For this review, take the finished solid that the model builds, in its own axes (mm). A direction names the side the tool comes from. Round coordinates to 2 decimals unless told otherwise and drop trailing zeros. Order: outer loops, then holes, each group sorted by start corner. A loop starts at its lowest first (then second) coordinate and runs counter-clockwise, first axis right, second up. Notation, with made-up numbers: (84.25, -17) -> (113.25, -17) arc R14 ccw to (113.25, -8) -> close; hole circle Ø7 at (76, -11). An arc over 180 degrees is marked (long way). Answer in a Markdown table with one row per item.
```python
from build123d import *

# Parameters (mm, degrees)
BOSS_EXTRUDE1_DEPTH = 2
SKETCH2_W           = 3
SKETCH2_H           = 52
BOSS_EXTRUDE2_DEPTH = 50
SKETCH3_R           = 4
CUT_EXTRUDE1_DEPTH  = 90


with BuildPart() as part:
    # Sketch1 → Boss-Extrude1 (new body)
    with BuildSketch(Plane(origin=(0, 0, 0), x_dir=(1, 0, 0), z_dir=(0, 1, 0))):
        with BuildLine():
            Line((-32.5, 28), (-27.204017471, 28))
            ThreePointArc((-27.204017471, 28), (-25.789803909, 27.414213562), (-25.204017471, 26))
            Line((-25.204017471, 26), (-25.204017471, -26))
            ThreePointArc((-25.204017471, -26), (-25.789803909, -27.414213562), (-27.204017471, -28))
            Line((-27.204017471, -28), (-32.5, -28))
            ThreePointArc((-32.5, -28), (-33.914213562, -28.585786438), (-34.5, -30))
            Line((-34.5, -30), (-34.5, -48))
            Line((-34.5, -48), (34.5, -48))
            Line((34.5, -48), (34.5, -30))
            ThreePointArc((34.5, -30), (33.914213562, -28.585786438), (32.5, -28))
            Line((32.5, -28), (27.204017471, -28))
            ThreePointArc((27.204017471, -28), (25.789803909, -27.414213562), (25.204017471, -26))
            Line((25.204017471, -26), (25.204017471, 26))
            ThreePointArc((25.204017471, 26), (25.789803909, 27.414213562), (27.204017471, 28))
            Line((27.204017471, 28), (32.5, 28))
            ThreePointArc((32.5, 28), (33.914213562, 28.585786438), (34.5, 30))
            Line((34.5, 30), (34.5, 48))
            Line((34.5, 48), (-34.5, 48))
            Line((-34.5, 48), (-34.5, 30))
            ThreePointArc((-34.5, 30), (-33.914213562, 28.585786438), (-32.5, 28))
        make_face()
        with BuildLine():
            Line((-26.353730012, 40.955917197), (-26.353730012, 38.634748977))
            ThreePointArc((-26.353730012, 38.634748977), (-27.768725827, 37.219753162), (-29.183721642, 38.634748977))
            Line((-29.183721642, 38.634748977), (-29.183721642, 40.955917197))
            ThreePointArc((-29.183721642, 40.955917197), (-27.768725827, 42.370913012), (-26.353730012, 40.955917197))
        make_face(mode=Mode.SUBTRACT)
        with BuildLine():
            Line((26.353730012, 40.955917197), (26.353730012, 38.634748977))
            ThreePointArc((26.353730012, 38.634748977), (27.768725827, 37.219753162), (29.183721642, 38.634748977))
            Line((29.183721642, 38.634748977), (29.183721642, 40.955917197))
            ThreePointArc((29.183721642, 40.955917197), (27.768725827, 42.370913012), (26.353730012, 40.955917197))
        make_face(mode=Mode.SUBTRACT)
        with BuildLine():
            Line((-26.353730012, -40.955917197), (-26.353730012, -38.634748977))
            ThreePointArc((-26.353730012, -38.634748977), (-27.768725827, -37.219753162), (-29.183721642, -38.634748977))
            Line((-29.183721642, -38.634748977), (-29.183721642, -40.955917197))
            ThreePointArc((-29.183721642, -40.955917197), (-27.768725827, -42.370913012), (-26.353730012, -40.955917197))
        make_face(mode=Mode.SUBTRACT)
        with BuildLine():
            Line((26.353730012, -40.955917197), (26.353730012, -38.634748977))
            ThreePointArc((26.353730012, -38.634748977), (27.768725827, -37.219753162), (29.183721642, -38.634748977))
            Line((29.183721642, -38.634748977), (29.183721642, -40.955917197))
            ThreePointArc((29.183721642, -40.955917197), (27.768725827, -42.370913012), (26.353730012, -40.955917197))
        make_face(mode=Mode.SUBTRACT)
    extrude(amount=BOSS_EXTRUDE1_DEPTH)

    # Sketch2 → Boss-Extrude2 (add)
    with BuildSketch(Plane(origin=(0, 2, 0), x_dir=(1, 0, 0), z_dir=(0, 1, 0))):
        with Locations((-23.704017471, 0)):
            Rectangle(SKETCH2_W, SKETCH2_H)
        with Locations((23.704017471, 0)):
            Rectangle(SKETCH2_W, SKETCH2_H)
    extrude(amount=BOSS_EXTRUDE2_DEPTH)

    # Sketch3 → Cut-Extrude1 (cut)
    with BuildSketch(Plane.ZY.offset(25.204017471)):
        with BuildLine():
            Line((-26, 52), (-26, 32))
            ThreePointArc((-26, 32), (-20.142135624, 46.142135624), (-6, 52))
            Line((-6, 52), (-26, 52))
        make_face()
        with BuildLine():
            ThreePointArc((6, 52), (20.142135624, 46.142135624), (26, 32))
            Line((26, 32), (26, 52))
            Line((26, 52), (6, 52))
        make_face()
        with Locations((0, 40)):
            Circle(SKETCH3_R)
    extrude(amount=-CUT_EXTRUDE1_DEPTH, mode=Mode.SUBTRACT)


solid = part.part
```
Q1. Take a section at C-C, the plane y = 40. Write out the cut boundary in (x, z), then the cut area to 3 significant figures.
Answer key:
| item | result |
|---|---|
| outline | (-25.2, -24.33) -> (-22.2, -24.33) -> (-22.2, -4) -> (-25.2, -4) -> close; (-25.2, 4) -> (-22.2, 4) -> (-22.2, 24.33) -> (-25.2, 24.33) -> close; (22.2, -24.33) -> (25.2, -24.33) -> (25.2, -4) -> (22.2, -4) -> close; (22.2, 4) -> (25.2, 4) -> (25.2, 24.33) -> (22.2, 24.33) -> close |
| area | 244 mm^2 |
Q2. Take a section at A-A, the plane z = 0. Write out the cut boundary in (x, y), then the cut area to 3 significant figures.
Answer key:
| item | result |
|---|---|
| outline | (-25.2, 0) -> (25.2, 0) -> (25.2, 36) -> (22.2, 36) -> (22.2, 2) -> (-22.2, 2) -> (-22.2, 36) -> (-25.2, 36) -> close; (-25.2, 44) -> (-22.2, 44) -> (-22.2, 52) -> (-25.2, 52) -> close; (22.2, 44) -> (25.2, 44) -> (25.2, 52) -> (22.2, 52) -> close |
| area | 353 mm^2 |
Q3. Clearance check with flat-ended pins moving along their axes: pin 1 Ø0.9 at (x, y) = (24, 11.5) entering from -Z; pin 2 Ø0.9 at (x, y) = (-23, 23) entering from +Z; pin 3 Ø12 at (x, z) = (-12, -19) entering from +Y; pin 4 Ø2 at (x, z) = (-27, 3.5) entering from -Y. State where each tip first meets the part, or that it passes through.
Answer key:
| item | result |
|---|---|
| pin 1 | stops at z = -26 |
| pin 2 | stops at z = 26 |
| pin 3 | stops at y = 2 |
| pin 4 | passes through |
Q4. The part is to be moulded in two halves that separate along X. For faces 1 (the face through (-30, 1, -28)), 2 (the face through (-27.8, 0.99, 42.37)), 3 (the face through (25.805, 0.986, 27.43)), say which applies: +X half, -X half, draft (parallel to the pull), parting line (faces both ways), or undercut.
Answer key:
| item | result |
|---|---|
| face 1 | draft |
| face 2 | undercut |
| face 3 | +X half |
Q5. Tool access review of faces 4 (the face through (29.184, 1, 40)), 5 (the face through (30, 1, 28)), 6 (the face through (-23.725, 46.297, 19.986)), 7 (the face through (-33.93, 0.99, -28.6)), 8 (the face through (-23.725, 43.966, -0.521)): name each direction out of +Z, -Z, +X, -X, +Y, -Y from which nothing blocks a thin tool from reaching the whole face with its end or side.
Answer key:
| item | result |
|---|---|
| face 4 | +Y, -Y |
| face 5 | +X, +Y, -Y |
| face 6 | +Z, +X, -X, +Y |
| face 7 | -X, +Y, -Y |
| face 8 | +X, -X |
Q6. Take a section at D-D, the plane z = 15. Write out the cut boundary in (x, y).
Answer key:
| item | result |
|---|---|
| outline | (-25.2, 0) -> (25.2, 0) -> (25.2, 49.86) -> (22.2, 49.86) -> (22.2, 2) -> (-22.2, 2) -> (-22.2, 49.86) -> (-25.2, 49.86) -> close |
Q7. Take a section at B-B, the plane y = 28. Write out the cut boundary in (x, z), then the cut area to 3 significant figures.
Answer key:
| item | result |
|---|---|
| outline | (-25.2, -26) -> (-22.2, -26) -> (-22.2, 26) -> (-25.2, 26) -> close; (22.2, -26) -> (25.2, -26) -> (25.2, 26) -> (22.2, 26) -> close |
| area | 312 mm^2 |
Q8. To check wall thickness, follow probe 1 along X at (y, z) = (49, -14); probe 2 along Y at (x, z) = (-24.4, 0); probe 3 along Y at (x, z) = (19.5, 11.5). State the ranges of each line that lie inside material, in increasing order.
Answer key:
| item | result |
|---|---|
| probe 1 | x = -25.2 to -22.2, 22.2 to 25.2 |
| probe 2 | y = 0 to 36, 44 to 52 |
| probe 3 | y = 0 to 2 |
